Work out the finished part from the listing and answer in its coordinate system (mm). Face numbers are marked on the shaded views. A direction names the side the tool comes from. Give positions to 0.01 mm unless a question says otherwise; leave off trailing zeros. Write each loop counter-clockwise with the first axis right and the second up, starting at its lowest first coordinate (ties: lowest second). Pieces come first, ordered by that corner, then holes. Notation, with made-up numbers: (54.5, 43) -> (100.5, 43) arc R22 ccw to (100.5, 72) -> close; hole circle Ø8 at (42.25, 53). An arc over 180 degrees is marked (long way). Write item = value, one per line. Start each with the question number.
from build123d import *

# Parameters (mm, degrees)
F1_DEPTH = 60
F2_R     = 50
F3_R     = 15
F4_T     = -2.5


with BuildPart() as f1:
    # F0 (on Top) → F1 (new body)
    with BuildSketch(Plane.XY):
        with BuildLine():
            Line((202.5, -202.5), (202.5, 0))
            ThreePointArc((202.5, 0), (0, 202.5), (-202.5, 0))
            Line((-202.5, 0), (-202.5, -202.5))
            Line((-202.5, -202.5), (202.5, -202.5))
        make_face()
    extrude(amount=F1_DEPTH)

    # F2
    f2_edges = [f1.edges().sort_by_distance(p)[0] for p in [
        (202.5, -202.5, 30),
        (-202.5, -202.5, 30),
    ]]
    fillet(f2_edges, radius=F2_R)

    # F3
    f3_edges = [f1.edges().sort_by_distance(p)[0] for p in [
        (-202.5, -76.25, 60),
        (-187.855339, -187.855339, 60),
        (0, 202.5, 60),
        (0, -202.5, 60),
        (202.5, -76.25, 60),
        (187.855339, -187.855339, 60),
    ]]
    fillet(f3_edges, radius=F3_R)

    # F4
    f4_openings = [f1.faces().sort_by_distance(p)[0] for p in [
        (0, -17.630456, 0),
    ]]
    offset(amount=F4_T, openings=f4_openings)


solid = f1.part
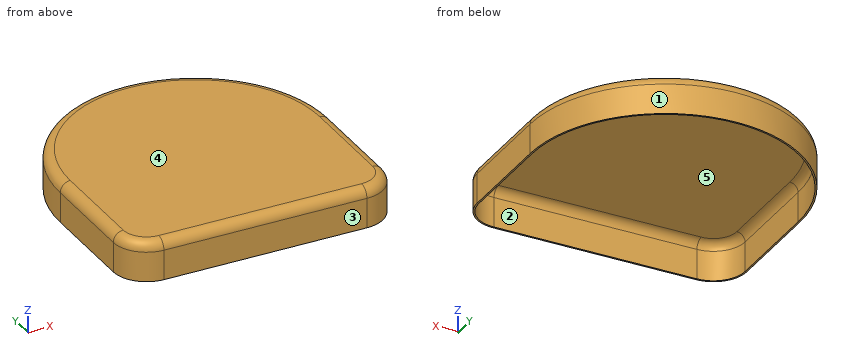
(1) For the marked faces 1 and 2, determine the directions among +Z, -Z, +X, -X, +Y, -Y from which every point of the face is accessible in a straight line to the end or side of a thin tool.
(2) Find the intervals of material crossed by line 1 along X through (y, z) = (-120, 10); line 2 along Z through (x, y) = (-36.5, 7); line 3 along Y through (x, z) = (-137, 9), in increasing order.
(3) Determine the mould class of the marked faces 3, 4 and 5 for opening direction Y: pulls with the +Y half, pulls with the -Y half, needs draft (parallel to the pull), parting line crosses it, or undercut.
(4) A cutting plane is placed at A-A, the plane z = 31. Write down the section's boundary in (x, y), then the cut area to 3 significant figures.
(5) A cutting plane is placed at B-B, the plane y = -26. Write down the section's boundary in (x, z), then the cut area to 3 significant figures.
(6) Each of these flat-tipped pins is pushed along its axis until it touches: pin 1 (3 mm diameter, centred on x = 95, y = 134.5, fed in from -Z); pin 2 (1 mm diameter, centred on y = 109.5, z = 28, fed in from -X); pin 3 (2 mm diameter, centred on x = -30.5, z = 53, fed in from -Y). Where does it stop, or does it pass through?
Results list:
q1.face_1 = +Z, -Z, +Y
q1.face_2 = -Z
q2.line_1 = -202.5 to -200, 200 to 202.5
q2.line_2 = 57.5 to 60
q2.line_3 = -202.5 to -200, 145.71 to 149.12
q3.face_3 = pulls with the -Y half
q3.face_4 = needs draft
q3.face_5 = undercut
q4.outline = (-202.5, -152.5) arc R50 ccw to (-152.5, -202.5) -> (152.5, -202.5) arc R50 ccw to (202.5, -152.5) -> (202.5, 0) arc R202.5 ccw to (-202.5, 0) -> close; hole (-200, -152.5) arc R47.5 ccw to (-152.5, -200) -> (152.5, -200) arc R47.5 ccw to (200, -152.5) -> (200, 0) arc R200 ccw to (-200, 0) -> close
q4.area = 3,490 mm²
q5.outline = (-202.5, 0) -> (-200, 0) -> (-200, 45) arc R12.5 cw to (-187.5, 57.5) -> (187.5, 57.5) arc R12.5 cw to (200, 45) -> (200, 0) -> (202.5, 0) -> (202.5, 45) arc R15 ccw to (187.5, 60) -> (-187.5, 60) arc R15 ccw to (-202.5, 45) -> close
q5.area = 1,270 mm²
q6.pin_1 = 57.5
q6.pin_2 = -170.66
q6.pin_3 = -200.77
